Work out the finished part from the listing and answer in its coordinate system (mm). Face numbers are marked on the shaded views. A direction names the side the tool comes from. Round coordinates to 2 decimals unless told otherwise and drop trailing zeros. Order: outer loops, then holes, each group sorted by start corner. A loop starts at its lowest first (then second) coordinate and runs counter-clockwise, first axis right, second up. Notation, with made-up numbers: (83.25, -39) -> (131.25, -39) arc R19 cw to (131.25, -8) -> close; hole circle Ø7 at (4, 72). An arc over 180 degrees is marked (long way). Use one line per item in the form item = value.
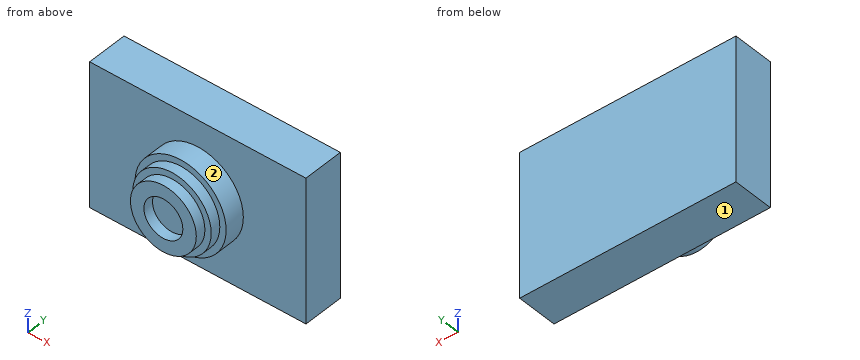
```python
from build123d import *

# Parameters (mm, degrees)
F0_W      = 135.262012
F0_H      = 90.036332
F1_DEPTH  = 25.4
F2_R      = 20.589532
F4_DEPTH  = 25.4
F3_R      = 10.44105
F5_DEPTH  = 38.1
F7_R      = 12.176484
F8_DEPTH  = 25.4
F9_R      = 24.533487
F10_DEPTH = 19.05
F11_R     = 28.476811
F12_DEPTH = 12.7


with BuildPart() as f1:
    # F0 (on Front) → F1 (new body)
    with BuildSketch(Plane.XZ):
        Rectangle(F0_W, F0_H)
    extrude(amount=F1_DEPTH)

    # F2 (on face) → F4 (join)
    with BuildSketch(Plane.XZ.offset(25.4)):
        Circle(F2_R)
    extrude(amount=F4_DEPTH)

    # F3 (on Front) → F5 (join)
    with BuildSketch(Plane.XZ):
        Circle(F3_R)
    extrude(amount=F5_DEPTH)

    # F7 (on face) → F8 (cut)
    with BuildSketch(Plane.XZ.offset(50.8)):
        Circle(F7_R)
    extrude(amount=-F8_DEPTH, mode=Mode.SUBTRACT)

    # F9 (on face) → F10 (join)
    with BuildSketch(Plane.XZ.offset(25.4)):
        Circle(F9_R)
    extrude(amount=F10_DEPTH)

    # F11 (on face) → F12 (join)
    with BuildSketch(Plane.XZ.offset(25.4)):
        Circle(F11_R)
    extrude(amount=F12_DEPTH)


solid = f1.part
```
Item 1: The part is cut by section A-A, the plane z = 0. Give the vertices of the cut face in (x, y), and give its area (3 significant figures).
Findings:
outline = (-67.63, -25.4) -> (-28.48, -25.4) -> (-28.48, -38.1) -> (-24.53, -38.1) -> (-24.53, -44.45) -> (-20.59, -44.45) -> (-20.59, -50.8) -> (-12.18, -50.8) -> (-12.18, -44.45) -> (12.18, -44.45) -> (12.18, -50.8) -> (20.59, -50.8) -> (20.59, -44.45) -> (24.53, -44.45) -> (24.53, -38.1) -> (28.48, -38.1) -> (28.48, -25.4) -> (67.63, -25.4) -> (67.63, 0) -> (-67.63, 0) -> close
area = 4,580 mm^2
Item 2: Flat-ended cylindrical pins translate along their axes: P1, Ø12, axis at x = -32, z = 15.5, coming from the -Y side; P2, Ø1.5, axis at y = -34, z = -24, coming from the +X side; P3, Ø1, axis at y = -42.5, z = -13, coming from the +X side. Find the tip coordinate at first contact, or state that the pin passes through.
Findings:
P1 = -25.4
P2 = 16.44
P3 = 21.11
Item 3: Consider line 1 along Z through (x, y) = (0, -49); line 2 along Y through (x, z) = (41, 2.5); line 3 along Z through (x, y) = (-1, -28). Determine where each line is inside the solid, lowest interval first.
Findings:
line_1 = -20.59 to -12.18, 12.18 to 20.59
line_2 = -25.4 to 0
line_3 = -28.46 to 28.46
Item 4: The part is cut by section C-C, the plane y = -40.5. Give the vertices of the cut face in (x, z), and give its area (3 significant figures).
Findings:
outline = circle Ø49.07 at (0, 0)
area = 1,890 mm^2
Item 5: For the marked faces 1 and 2, determine the directions among +Z, -Z, +X, -X, +Y, -Y from which every point of the face is accessible in a straight line to the end or side of a thin tool.
Findings:
face_1 = -Z, +X, -X, +Y, -Y
face_2 = -Y
Item 6: The part is cut by section B-B, the plane x = -4.5. Give the vertices of the cut face in (y, z).
Findings:
outline = (-50.8, -20.09) -> (-44.45, -20.09) -> (-44.45, -24.12) -> (-38.1, -24.12) -> (-38.1, -28.12) -> (-25.4, -28.12) -> (-25.4, -45.02) -> (0, -45.02) -> (0, 45.02) -> (-25.4, 45.02) -> (-25.4, 28.12) -> (-38.1, 28.12) -> (-38.1, 24.12) -> (-44.45, 24.12) -> (-44.45, 20.09) -> (-50.8, 20.09) -> (-50.8, 11.31) -> (-44.45, 11.31) -> (-44.45, -11.31) -> (-50.8, -11.31) -> close
Item 7: The part is cut by section D-D, the plane z = 33. Give the vertices of the cut face in (x, y), and give its area (3 significant figures).
Findings:
outline = (-67.63, -25.4) -> (67.63, -25.4) -> (67.63, 0) -> (-67.63, 0) -> close
area = 3,440 mm^2
